Drawing for the job (mm, zero at the part's lowest x, y, z). A direction names the side the tool comes from. Round coordinates to 2 decimals unless told otherwise and drop trailing zeros. Loops run counter-clockwise (first coordinate to the right, second up) from the corner with the lowest first, then second, coordinate; pieces in that order, holes last. Notation, with made-up numbers: (60.5, 51) -> (93.5, 51) arc R25 ccw to (93.5, 73) -> close; hole circle Ø1 at (-35, -14). An arc over 180 degrees is marked (long way). Put each result on its own line as item: value. Start each with the question number.
Item 1: Cut at C-C, the plane z = 2.1. List the corners of the cut face in (x, y).
Item 2: Cut at B-B, the plane x = 3.15. List the corners of the cut face in (y, z), plus the area to 3 significant figures.
Item 3: Tool access for the marked faces 4 and 5: list every direction of +Z, -Z, +X, -X, +Y, -Y with a clear straight run to the whole face (end or side of a thin tool).
Item 4: Flat gauge pins, fed straight in: pin 1 Ø2 at (x, z) = (3, 4) entering from -Y; pin 2 Ø0.6 at (x, y) = (1.5, 3.5) entering from +Z; pin 3 Ø1.8 at (x, y) = (9.65, 5.7) entering from -Z; pin 4 Ø0.8 at (x, y) = (1, 2) entering from -Z. Where does each tip first touch, or does it go through?
Item 5: Cut at D-D, the plane y = 1.25. List the corners of the cut face in (x, z).
Item 6: Pull direction Y, two halves, no side cores. Call the marked faces 1, 2 and 3: +Y half, -Y half, draft (parallel to the pull), parting line (faces both ways), or undercut.
Item 7: Cut at A-A, the plane y = 5.7. List the corners of the cut face in (x, z), plus the area to 3 significant figures.
Item 8: Drill centre lines: probe 1 along X at (y, z) = (2.25, 2.75); probe 2 along Y at (x, z) = (3.15, 1.55); probe 3 along Y at (x, z) = (8.25, 3.85). Where is each one in solid material? Low to high. Write a range as [from, to].
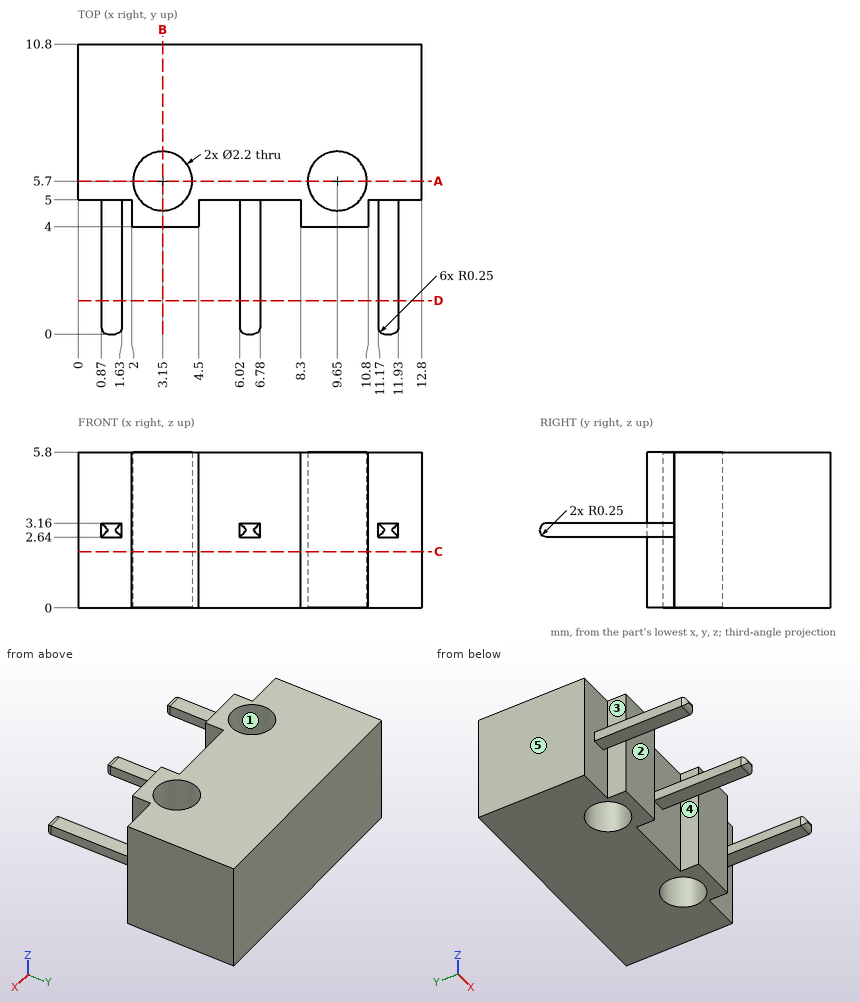
Reply:
1. outline: (0, 5) -> (2, 5) -> (2, 4) -> (4.5, 4) -> (4.5, 5) -> (8.3, 5) -> (8.3, 4) -> (10.8, 4) -> (10.8, 5) -> (12.8, 5) -> (12.8, 10.8) -> (0, 10.8) -> close; hole circle Ø2.2 at (3.15, 5.7); hole circle Ø2.2 at (9.65, 5.7)
2. outline: (4, 0) -> (4.6, 0) -> (4.6, 5.8) -> (4, 5.8) -> close; (6.8, 0) -> (10.8, 0) -> (10.8, 5.8) -> (6.8, 5.8) -> close
2. area: 26.7 mm^2
3. face 4: +Z, -Z, -Y
3. face 5: +Z, -Z, -X, +Y, -Y
4. pin 1: stops at y = 4
4. pin 2: stops at z = 3.16
4. pin 3: passes through
4. pin 4: stops at z = 2.64
5. outline: (0.87, 2.64) -> (1.63, 2.64) -> (1.63, 3.16) -> (0.87, 3.16) -> close; (6.02, 2.64) -> (6.78, 2.64) -> (6.78, 3.16) -> (6.02, 3.16) -> close; (11.17, 2.64) -> (11.93, 2.64) -> (11.93, 3.16) -> (11.17, 3.16) -> close
6. face 1: undercut
6. face 2: -Y half
6. face 3: draft
7. outline: (0, 0) -> (2.05, 0) -> (2.05, 5.8) -> (0, 5.8) -> close; (4.25, 0) -> (8.55, 0) -> (8.55, 5.8) -> (4.25, 5.8) -> close; (10.75, 0) -> (12.8, 0) -> (12.8, 5.8) -> (10.75, 5.8) -> close
7. area: 48.7 mm^2
8. probe 1: x = [0.87, 1.63], [6.02, 6.78], [11.17, 11.93]
8. probe 2: y = [4, 4.6], [6.8, 10.8]
8. probe 3: y = [5, 10.8]
